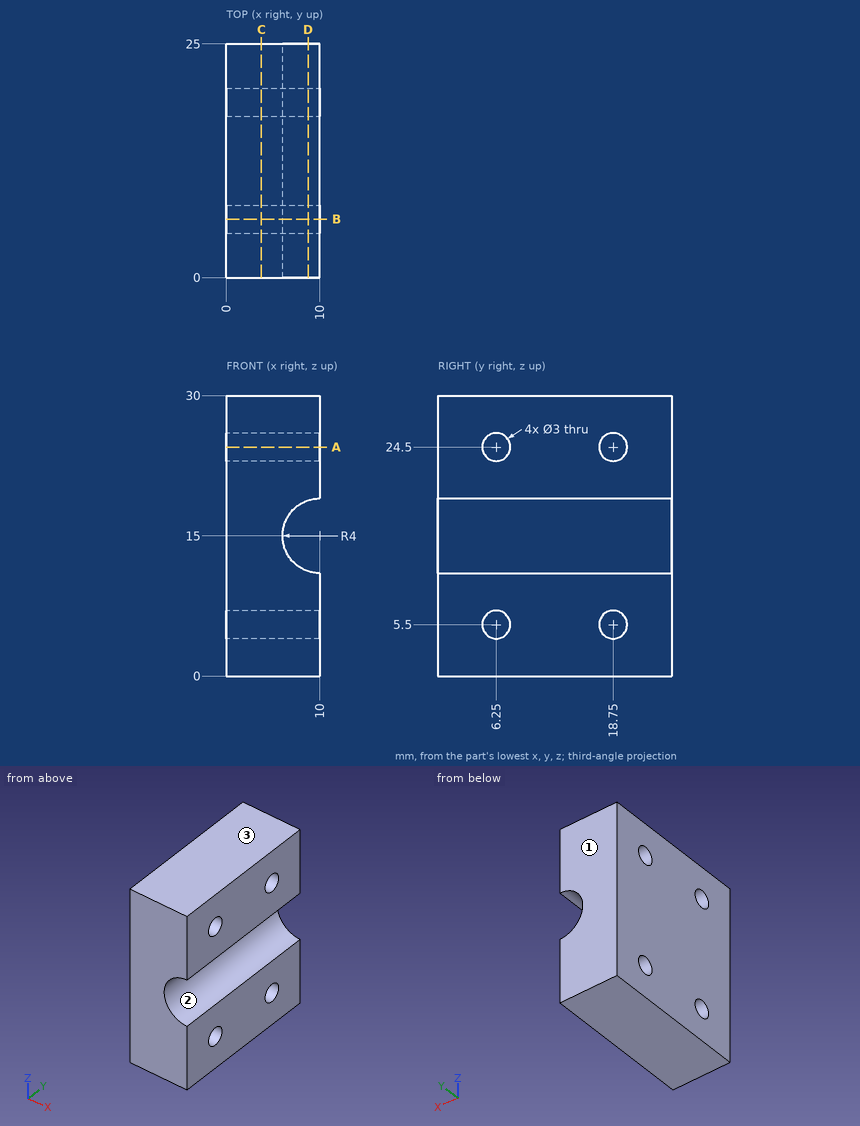
For this review, use the dimensioned drawing (mm, ordinates from the lowest corner) and the shaded views. Give positions to 0.01 mm unless a question says otherwise; leave off trailing zeros. Order: outer loops, then holes, each group sorted by start corner. A loop starts at its lowest first (then second) coordinate and runs counter-clockwise, first axis right, second up. Notation, with made-up numbers: (75, 15.25) -> (128, 15.25) arc R15 ccw to (128, 31.25) -> close; hole circle Ø7 at (23, 32.5). An arc over 180 degrees is marked (long way). Write item = value, one per line. Start each with the question number.
(1) Take a section at B-B (y = 6.25). Write out the cut boundary in (x, z).
(2) Take a section at A-A (z = 24.5). Write out the cut boundary in (x, y).
(3) Take a section at C-C (x = 3.75). Write out the cut boundary in (y, z), plus the area to 3 significant figures.
(4) For pin 1 Ø1.8 at (y, z) = (18.75, 5.5) entering from -X, flat-tipped, find the tip position at first contact; note if it passes through.
(5) Take a section at D-D (x = 8.75). Write out the cut boundary in (y, z), plus the area to 3 significant figures.
(6) Draft analysis for pull direction Z (two halves, no side actions). For the marked faces 1, 2 and 3, state which applies: +Z half, -Z half, draft (parallel to the pull), parting line (faces both ways), or undercut.
(7) For L1, parallel to Y at x = 6, z = 5.5; L2, parallel to Z at x = 8.75, y = 5.75; L3, parallel to Z at x = 8.75, y = 17.75, list the stretches that pass through material, from the lowest coordinate up. Write a range as from..to.
Returned:
q1.outline = (0, 0) -> (10, 0) -> (10, 4) -> (0, 4) -> close; (0, 7) -> (10, 7) -> (10, 11) arc R4 cw to (10, 19) -> (10, 23) -> (0, 23) -> close; (0, 26) -> (10, 26) -> (10, 30) -> (0, 30) -> close
q2.outline = (0, 0) -> (10, 0) -> (10, 4.75) -> (0, 4.75) -> close; (0, 7.75) -> (10, 7.75) -> (10, 17.25) -> (0, 17.25) -> close; (0, 20.25) -> (10, 20.25) -> (10, 25) -> (0, 25) -> close
q3.outline = (0, 0) -> (25, 0) -> (25, 30) -> (0, 30) -> close; hole circle Ø3 at (6.25, 5.5); hole circle Ø3 at (6.25, 24.5); hole circle Ø3 at (18.75, 5.5); hole circle Ø3 at (18.75, 24.5)
q3.area = 722 mm²
q4.pin_1 = through
q5.outline = (0, 0) -> (25, 0) -> (25, 11.2) -> (0, 11.2) -> close; (0, 18.8) -> (25, 18.8) -> (25, 30) -> (0, 30) -> close; hole circle Ø3 at (6.25, 5.5); hole circle Ø3 at (6.25, 24.5); hole circle Ø3 at (18.75, 5.5); hole circle Ø3 at (18.75, 24.5)
q5.area = 532 mm²
q6.face_1 = draft
q6.face_2 = undercut
q6.face_3 = +Z half
q7.L1 = 0..4.75, 7.75..17.25, 20.25..25
q7.L2 = 0..4.09, 6.91..11.2, 18.8..23.09, 25.91..30
q7.L3 = 0..4.38, 6.62..11.2, 18.8..23.38, 25.62..30
